from build123d import *

# Parameters (mm, degrees)
SKETCH10_R                = 1
BOSS_EXTRUDE5_DEPTH       = 7.5
CUT_EXTRUDE1_DEPTH        = 4
FILLET1_R                 = 10
CUT_EXTRUDE6_START        = -11
CUT_EXTRUDE6_DEPTH        = 10
CUT_EXTRUDE7_DEPTH        = 2
BOSS_EXTRUDE11_DEPTH      = 9
SKETCH28_R                = 1
CUT_EXTRUDE8_DEPTH        = 9
BOSS_EXTRUDE13_DEPTH      = 80
BOSS_EXTRUDE13_DEPTH_BACK = 3
SKETCH30_W                = 2
SKETCH30_H                = 15
BOSS_EXTRUDE14_DEPTH      = 14
BOSS_EXTRUDE14_DEPTH_BACK = 4
SKETCH31_W                = 1.5
SKETCH31_H                = 29.5
SKETCH31_W_2              = 0.5
SKETCH31_H_2              = 3.0862264
CUT_EXTRUDE9_DEPTH        = 9
FILLET2_R                 = 8
FILLET3_R                 = 10
BOSS_EXTRUDE15_DEPTH      = 2
BOSS_EXTRUDE16_START      = 2
BOSS_EXTRUDE16_DEPTH      = 2


with BuildPart() as part:
    # Sketch10 → Boss-Extrude5 (new, symmetric)
    with BuildSketch(Plane.XY):
        Polygon((27.048887868, 48.656944563), (33.959433176, 37.989988632), (36.993816658, 26.682834617), (12.788755024, 23.658848526), (10.279677841, 36.875809012), (12.321789019, 48.656944563), align=None)
        with Locations((17.890076876, 43.12952492)):
            Circle(SKETCH10_R, mode=Mode.SUBTRACT)
        with Locations((23.882298789, 39.668364252)):
            Circle(SKETCH10_R, mode=Mode.SUBTRACT)
    extrude(amount=BOSS_EXTRUDE5_DEPTH, both=True)

    # Sketch11 → Cut-Extrude1 (cut)
    with BuildSketch(Plane.XY.offset(7.5)):
        with BuildLine():
            Line((17.825431655, 32.423947427), (9.123881611, 30.207909529))
            Line((9.123881611, 30.207909529), (6.594316119, 53.15991455))
            Line((6.594316119, 53.15991455), (34.693470887, 60.271659822))
            Line((34.693470887, 60.271659822), (37.752907488, 30.846026516))
            add(Edge.make_bspline(
                [(37.752907488, 30.846026516), (30.679137573, 30.15507536), (19.269012528, 26.734198276), (17.825431655, 32.423947427)],
                knots=[0, 0, 0, 0, 1, 1, 1, 1], degree=3))
        make_face()
    extrude(amount=-CUT_EXTRUDE1_DEPTH, mode=Mode.SUBTRACT)

    # Fillet1
    fillet1_edges = [part.edges().sort_by_distance(p)[0] for p in [
        (27.048887868, 48.656944563, -2),
    ]]
    fillet(fillet1_edges, radius=FILLET1_R)

    # Sketch11_2 → Cut-Extrude6 (cut)
    with BuildSketch(Plane.XY.offset(7.5).offset(CUT_EXTRUDE6_START)):
        with BuildLine():
            Line((17.825431655, 32.423947427), (9.123881611, 30.207909529))
            Line((9.123881611, 30.207909529), (6.594316119, 53.15991455))
            Line((6.594316119, 53.15991455), (34.693470887, 60.271659822))
            Line((34.693470887, 60.271659822), (37.752907488, 30.846026516))
            add(Edge.make_bspline(
                [(37.752907488, 30.846026516), (30.679137573, 30.15507536), (19.269012528, 26.734198276), (17.825431655, 32.423947427)],
                knots=[0, 0, 0, 0, 1, 1, 1, 1], degree=3))
        make_face()
    extrude(amount=-CUT_EXTRUDE6_DEPTH, mode=Mode.SUBTRACT)

    # Sketch16 → Cut-Extrude7 (cut, symmetric)
    with BuildSketch(Plane.XY):
        Polygon((10.074284509, 54.36084815), (34.418624568, 54.36084815), (34.418624568, 36.664364271), (10.074284509, 40.645108775), align=None)
    extrude(amount=CUT_EXTRUDE7_DEPTH, both=True, mode=Mode.SUBTRACT)

    # Sketch26 → Boss-Extrude11 (add)
    with BuildSketch(Plane(origin=(41.188168375, 11.053240949, 0), x_dir=(0, 0, -1), z_dir=(0.9658266565657433, 0.2591888683316433, 0))):
        Polygon((2, 27.88983665), (2, 26.535626274), (-2, 26.535626274), (-2, 27.88983665), (-3.5, 27.88983665), (-3.5, 20.267140373), (-7.5, 20.267140373), (-7.5, 16.182607471), (7.5, 16.182607471), (7.5, 20.267140372), (3.5, 20.267140373), (3.5, 27.88983665), align=None)
    extrude(amount=BOSS_EXTRUDE11_DEPTH)

    # Sketch28 → Cut-Extrude8 (cut)
    with BuildSketch(Plane(origin=(-4.194351717, 15.629593668, 0), x_dir=(0.9658266565657433, 0.25918886833164334, 0), z_dir=(0.25918886833164334, -0.9658266565657433, 0))):
        with Locations((38.244135106, 4.615132599)):
            Circle(SKETCH28_R)
        with Locations((38.244135106, -4.615132599)):
            Circle(SKETCH28_R)
    extrude(amount=-CUT_EXTRUDE8_DEPTH, mode=Mode.SUBTRACT)

    # Sketch30 → Boss-Extrude13 (add, two sides: drawn at the far end of the back side and taken through both)
    with BuildSketch(Plane(origin=(-4.194351717, 15.629593668, 0), x_dir=(0.9658266565657433, 0.25918886833164334, 0), z_dir=(0.25918886833164334, -0.9658266565657433, 0)).offset(-BOSS_EXTRUDE13_DEPTH_BACK)):
        with Locations((27.645507965, 0)):
            Rectangle(SKETCH30_W, SKETCH30_H)
        with Locations((25.645507965, 0)):
            Rectangle(SKETCH30_W, SKETCH30_H)
    extrude(amount=BOSS_EXTRUDE13_DEPTH + BOSS_EXTRUDE13_DEPTH_BACK)

    # Sketch31 → Boss-Extrude14 (add, two sides: drawn at the far end of the back side and taken through both)
    with BuildSketch(Plane(origin=(27.666595183, 7.424596792, 0), x_dir=(0, 0, -1), z_dir=(0.9658266565657432, 0.2591888683316434, 0)).offset(-BOSS_EXTRUDE14_DEPTH_BACK)):
        with Locations((-6.75, -48.567392529)):
            Rectangle(SKETCH31_W, SKETCH31_H)
        with Locations((-7.75, -48.567392529)):
            Rectangle(SKETCH31_W_2, SKETCH31_H)
        with Locations((6.75, -48.567392529)):
            Rectangle(SKETCH31_W, SKETCH31_H)
        with Locations((7.75, -48.567392529)):
            Rectangle(SKETCH31_W_2, SKETCH31_H)
        Polygon((-3, -63.317392529), (-6, -63.317392529), (-7.5, -63.317392529), (-7.5, -63.817392529), (-3, -63.817392529), align=None)
        Polygon((7.5, -63.817392529), (3, -63.817392529), (3, -65.317392529), (8, -65.317392529), (8, -63.317392529), (7.5, -63.317392529), align=None)
        Polygon((3, -63.317392529), (3, -63.817392529), (7.5, -63.817392529), (7.5, -63.317392529), (6, -63.317392529), align=None)
        Polygon((-7.5, -63.817392529), (-7.5, -63.317392529), (-8, -63.317392529), (-8, -65.317392529), (-3, -65.317392529), (-3, -63.817392529), align=None)
        Polygon((-7.5, -33.817392529), (-6, -33.817392529), (-3.25, -33.817392529), (-3.25, -30.731166129), (-7.5, -30.731166129), align=None)
        Polygon((3.25, -33.817392529), (6, -33.817392529), (7.5, -33.817392529), (7.5, -30.731166129), (3.25, -30.731166129), align=None)
        with Locations((7.75, -32.274279329)):
            Rectangle(SKETCH31_W_2, SKETCH31_H_2)
        with Locations((-7.75, -32.274279329)):
            Rectangle(SKETCH31_W_2, SKETCH31_H_2)
    extrude(amount=BOSS_EXTRUDE14_DEPTH + BOSS_EXTRUDE14_DEPTH_BACK)

    # Sketch32 → Cut-Extrude9 (cut)
    with BuildSketch(Plane(origin=(49.880608284, 13.385940764, 0), x_dir=(0, 0, -1), z_dir=(0.9658266565657431, 0.25918886833164445, 0))):
        Polygon((3.5, 27.88983665), (2, 27.88983665), (2, 26.535626274), (-2, 26.535626274), (-2, 27.88983665), (-3.5, 27.88983665), (-3.5, 20.267140373), (-7.5, 20.267140373), (-7.5, 16.182607471), (7.5, 16.182607471), (7.5, 20.267140372), (3.5, 20.267140373), align=None)
    extrude(amount=-CUT_EXTRUDE9_DEPTH, mode=Mode.SUBTRACT)

    # Fillet2
    fillet2_edges = [part.edges().sort_by_distance(p)[0] for p in [
        (12.321789019, 48.656944563, 2.75),
        (12.321789019, 48.656944563, -2.75),
    ]]
    fillet(fillet2_edges, radius=FILLET2_R)

    # Fillet3
    fillet3_edges = [part.edges().sort_by_distance(p)[0] for p in [
        (17.825431655, 32.423947427, 5.5),
        (17.825431655, 32.423947427, -5.5),
    ]]
    fillet(fillet3_edges, radius=FILLET3_R)

    # Sketch33 → Boss-Extrude15 (add)
    with BuildSketch(Plane(origin=(0, 0, -7.5), x_dir=(-1, 0, 0), z_dir=(0, 0, -1))):
        with BuildLine():
            Line((-11.433819556, 30.796185182), (-12.326379112, 31.023494775))
            ThreePointArc((-12.326379112, 31.023494775), (-16.080268918, 31.249787506), (-19.652288318, 30.073533078))
            add(Edge.make_bspline(
                [(-19.652288318, 30.073533078), (-23.094178016, 28.160579122), (-30.349802092, 29.858629099), (-35.935151197, 30.627785373)],
                knots=[0.191604014, 0.191604014, 0.191604014, 0.191604014, 0.918085752, 0.918085752, 0.918085752, 0.918085752], degree=3))
            Line((-35.935151197, 30.627785373), (-36.993816658, 26.682834617))
            Line((-36.993816658, 26.682834617), (-22.968678464, 24.93064644))
            Line((-22.968678464, 24.93064644), (-12.788755024, 23.658848526))
            Line((-12.788755024, 23.658848526), (-11.433819556, 30.796185182))
        make_face()
    extrude(amount=BOSS_EXTRUDE15_DEPTH)

    # Sketch34 → Boss-Extrude16 (add)
    with BuildSketch(Plane.XY.offset(7.5).offset(BOSS_EXTRUDE16_START)):
        with BuildLine():
            Line((12.326379112, 31.023494775), (11.433819556, 30.796185182))
            Line((11.433819556, 30.796185182), (12.788755024, 23.658848526))
            Line((12.788755024, 23.658848526), (22.968678464, 24.93064644))
            Line((22.968678464, 24.93064644), (36.993816658, 26.682834617))
            Line((36.993816658, 26.682834617), (35.935151197, 30.627785373))
            add(Edge.make_bspline(
                [(35.935151197, 30.627785373), (30.349802091, 29.858629099), (23.094178016, 28.160579122), (19.652288318, 30.073533078)],
                knots=[0.191604014, 0.191604014, 0.191604014, 0.191604014, 0.918085752, 0.918085752, 0.918085752, 0.918085752], degree=3))
            ThreePointArc((19.652288318, 30.073533078), (16.080268918, 31.249787506), (12.326379112, 31.023494775))
        make_face()
    extrude(amount=-BOSS_EXTRUDE16_DEPTH)


solid = part.part
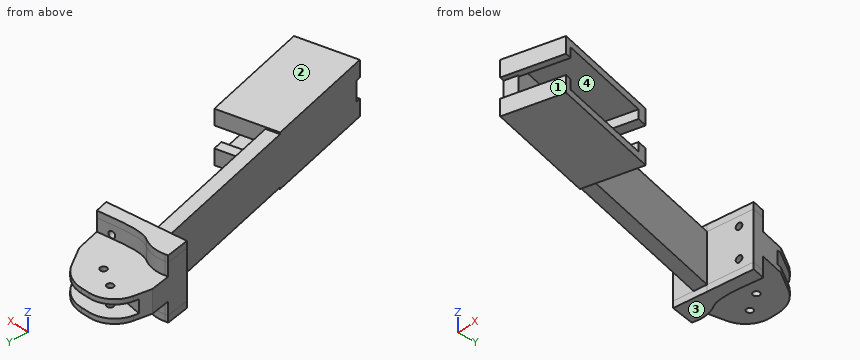
Source: CAD feature listing. Evaluate the final solid. Frame: model axes, mm. Face numbers are marked on the shaded views. Coordinates: 2 decimals unless noted, no trailing zeros. Loops run counter-clockwise (first coordinate to the right, second up) from the corner with the lowest first, then second, coordinate; pieces in that order, holes last. Notation, with made-up numbers: (79.5, 34) -> (89.5, 34) arc R21 ccw to (89.5, 64) -> close; hole circle Ø1 at (36.5, 89). An arc over 180 degrees is marked (long way). Answer in a Markdown table with one row per item. Add a question column.
Q1. Pull-direction query (Z, two-part tool) for the marked faces 1, 2, 3 and 4; classes: pulls with the +Z half, pulls with the -Z half, needs draft (parallel to the pull), parting line crosses it, or undercut.
Q2. Section A-A on z = 0.5. Return the cut outline in (x, y), and give its area (3 significant figures).
Q3. Section C-C on x = 39. Return the cut outline in (y, z), and give its area (3 significant figures).
Q4. Section D-D on y = -6. Return the cut outline in (x, z).
Q5. Contact query for flat-ended pins moving along their axis: pin 1 Ø2.5 at (x, y) = (23.88, 39.67) entering from -Z; pin 2 Ø3.5 at (x, y) = (49.5, -52.5) entering from -Z; pin 3 Ø2 at (x, z) = (50, -4) entering from -Y. Output: stop coordinate, or through.
Q6. Ray query, line 1 along Z through (x, y) = (52, -35.5); line 2 along Z through (x, y) = (38, -23.5); line 3 along Z through (x, y) = (26.5, 3). Return the intervals inside material, ascending.
Q7. Section B-B on x = 52.5. Return the cut outline in (y, z), and give its area (3 significant figures).
Computed values:
| question | item | result |
|---|---|---|
| 1 | face 1 | needs draft |
| 1 | face 2 | pulls with the +Z half |
| 1 | face 3 | pulls with the -Z half |
| 1 | face 4 | undercut |
| 2 | outline | (10.28, 36.88) -> (12.79, 23.66) -> (18.96, 24.43) -> (40.34, -55.25) -> (44.21, -54.21) -> (22.97, 24.93) -> (36.99, 26.68) -> (34.31, 36.68) -> (10.91, 40.51) -> close |
| 2 | area | 656 mm^2 |
| 3 | outline | (-50.24, -8) -> (-21.35, -8) -> (-21.35, -3.25) -> (-24.55, -3.25) -> (-24.55, -6) -> (-34.81, -6) -> (-34.81, 6) -> (-24.55, 6) -> (-24.55, 3.25) -> (-21.35, 3.25) -> (-21.35, 8) -> (-50.24, 8) -> close |
| 3 | area | 318 mm^2 |
| 4 | outline | (27.13, -7.5) -> (31.27, -7.5) -> (31.27, 7.5) -> (27.13, 7.5) -> close |
| 5 | pin 1 | stops at z = -3.5 |
| 5 | pin 2 | stops at z = -8 |
| 5 | pin 3 | stops at y = -54.48 |
| 6 | line 1 | z = -8 to -6, 6 to 8 |
| 6 | line 2 | z = -8 to -3.25, 3.25 to 8 |
| 6 | line 3 | z = -7.5 to 7.5 |
| 7 | outline | (-53.54, -8) -> (-31.1, -8) -> (-31.1, -6) -> (-51.47, -6) -> (-51.47, -3) -> (-53.54, -3) -> close; (-53.54, 3) -> (-51.47, 3) -> (-51.47, 6) -> (-31.1, 6) -> (-31.1, 8) -> (-53.54, 8) -> close |
| 7 | area | 102 mm^2 |
